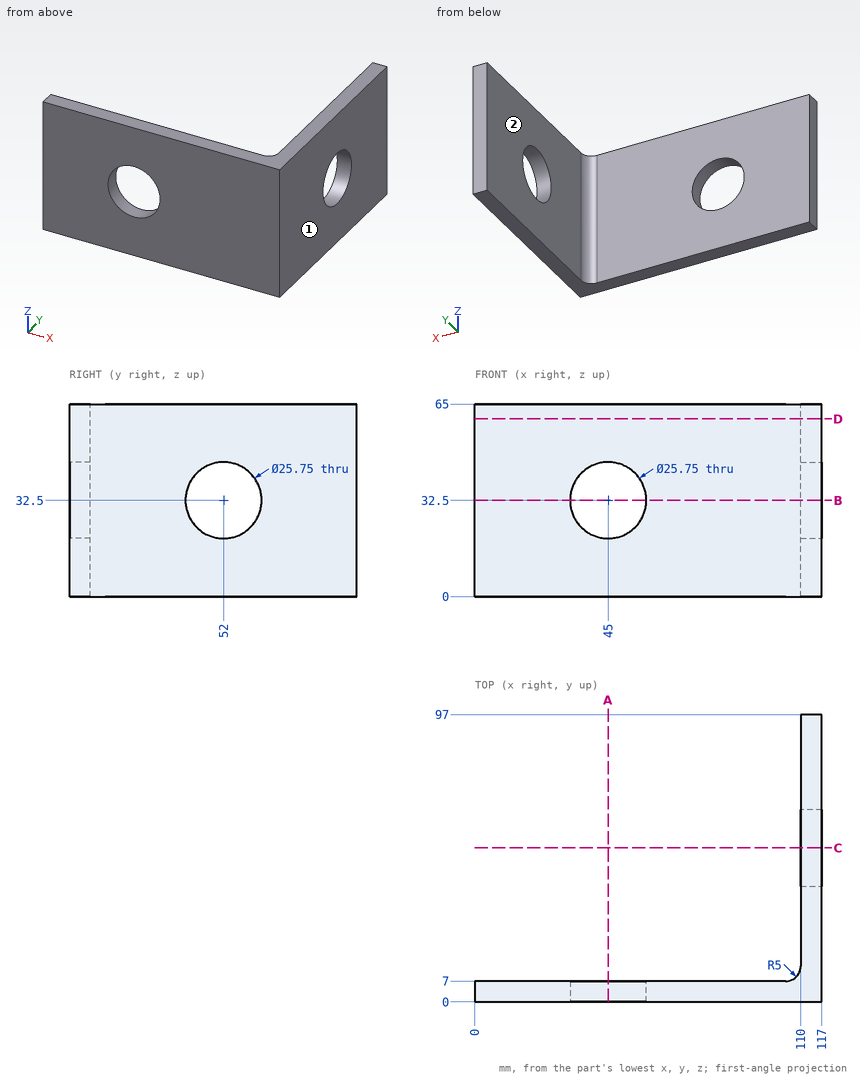
Part print with two shaded views. Sizes in mm from the minimum x, y, z corner. A direction names the side the tool comes from. Round coordinates to 2 decimals unless told otherwise and drop trailing zeros. Loops run counter-clockwise (first coordinate to the right, second up) from the corner with the lowest first, then second, coordinate; pieces in that order, holes last. Notation, with made-up numbers: (-12, 62.25) - (25, 62.25) arc R34 ccw to (25, 101.25) - close; hole circle Ø6 at (7, 6). An arc over 180 degrees is marked (long way). Answer as a JSON object with one key per item and string values.
Item 1: Band-saw the part on C-C on y = 52. List the corners of the cut face in (x, z) (3 decimals), plus the area to 3 significant figures.
Output:
{"outline": "(110, 0) - (117, 0) - (117, 19.625) - (110, 19.625) - close; (110, 45.375) - (117, 45.375) - (117, 65) - (110, 65) - close", "area": "275 mm2"}
Item 2: Band-saw the part on D-D on z = 60. List the corners of the cut face in (x, y).
Output:
{"outline": "(0, 0) - (117, 0) - (117, 97) - (110, 97) - (110, 12) arc R5 cw to (105, 7) - (0, 7) - close"}
Item 3: Band-saw the part on A-A on x = 45. List the corners of the cut face in (y, z) (3 decimals).
Output:
{"outline": "(0, 0) - (7, 0) - (7, 19.625) - (0, 19.625) - close; (0, 45.375) - (7, 45.375) - (7, 65) - (0, 65) - close"}
Item 4: Band-saw the part on B-B on z = 32.5. List the corners of the cut face in (x, y) (3 decimals), plus the area to 3 significant figures.
Output:
{"outline": "(0, 0) - (32.125, 0) - (32.125, 7) - (0, 7) - close; (57.875, 0) - (117, 0) - (117, 39.125) - (110, 39.125) - (110, 12) arc R5 cw to (105, 7) - (57.875, 7) - close; (110, 64.875) - (117, 64.875) - (117, 97) - (110, 97) - close", "area": "1,090 mm2"}
Item 5: Wall check: L1, parallel to Z at x = 45, y = 3.75 (3 decimals); L2, parallel to Y at x = 99, z = 34.5; L3, parallel to X at y = 70, z = 42. Give the ranges that are in metal, low to high.
Output:
{"L1": "0 to 19.625, 45.375 to 65", "L2": "0 to 7", "L3": "110 to 117"}
Item 6: Tool access for the marked faces 1 and 2: list every direction of +Z, -Z, +X, -X, +Y, -Y with a clear straight run to the whole face (end or side of a thin tool).
Output:
{"face 1": "+Z, -Z, +X, +Y, -Y", "face 2": "+Z, -Z, -X, +Y"}
Item 7: Pin check, flat tips, straight feed: pin 1 (3 mm diameter, centred on y = 23, z = 19.5, fed in from -X); pin 2 (1 mm diameter, centred on x = 12.5, z = 31, fed in from -Y); pin 3 (5 mm diameter, centred on x = 94, z = 48, fed in from +Y). Stop position of each tip, or through.
Output:
{"pin 1": "x = 110", "pin 2": "y = 0", "pin 3": "y = 7"}
